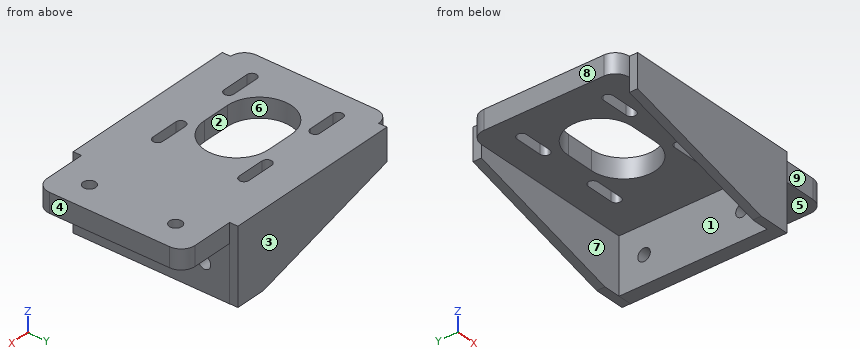
from build123d import *

# Parameters (mm, degrees)
F0_W      = 90
F0_H      = 53.2
F0_R      = 2.25
F1_DEPTH  = 3.5
F2_R      = 5
F3_W      = 5
F3_H      = 20
F4_DEPTH  = 26.6
F6_DEPTH  = 3
F8_DEPTH  = 3
F9_R      = 2.25
F10_DEPTH = 5


with BuildPart() as f1:
    # F0 (on Top) → F1 (new body, symmetric)
    with BuildSketch(Plane.XY):
        Rectangle(F0_W, F0_H)
        with BuildLine():
            ThreePointArc((-35.77, -17.25), (-37.52, -15.5), (-35.77, -13.75))
            Line((-35.77, -13.75), (-25.77, -13.75))
            ThreePointArc((-25.77, -13.75), (-24.02, -15.5), (-25.77, -17.25))
            Line((-25.77, -17.25), (-35.77, -17.25))
        make_face(mode=Mode.SUBTRACT)
        with BuildLine():
            Line((-4.77, -13.75), (5.23, -13.75))
            ThreePointArc((5.23, -13.75), (6.98, -15.5), (5.23, -17.25))
            Line((5.23, -17.25), (-4.77, -17.25))
            ThreePointArc((-4.77, -17.25), (-6.52, -15.5), (-4.77, -13.75))
        make_face(mode=Mode.SUBTRACT)
        with Locations((35, -15.5)):
            Circle(F0_R, mode=Mode.SUBTRACT)
        with BuildLine():
            ThreePointArc((-10.27, 11.5), (1.23, 0), (-10.27, -11.5))
            Line((-10.27, -11.5), (-20.27, -11.5))
            ThreePointArc((-20.27, -11.5), (-31.77, 0), (-20.27, 11.5))
            Line((-20.27, 11.5), (-10.27, 11.5))
        make_face(mode=Mode.SUBTRACT)
        with BuildLine():
            Line((-25.77, 13.75), (-35.77, 13.75))
            ThreePointArc((-35.77, 13.75), (-37.52, 15.5), (-35.77, 17.25))
            Line((-35.77, 17.25), (-25.77, 17.25))
            ThreePointArc((-25.77, 17.25), (-24.02, 15.5), (-25.77, 13.75))
        make_face(mode=Mode.SUBTRACT)
        with BuildLine():
            ThreePointArc((5.23, 17.25), (6.98, 15.5), (5.23, 13.75))
            Line((5.23, 13.75), (-4.77, 13.75))
            ThreePointArc((-4.77, 13.75), (-6.52, 15.5), (-4.77, 17.25))
            Line((-4.77, 17.25), (5.23, 17.25))
        make_face(mode=Mode.SUBTRACT)
        with Locations((35, 15.5)):
            Circle(F0_R, mode=Mode.SUBTRACT)
    extrude(amount=F1_DEPTH, both=True)

    # F2
    f2_edges = [f1.edges().sort_by_distance(p)[0] for p in [
        (-45, 26.6, 0),
        (-45, -26.6, 0),
        (45, -26.6, 0),
        (45, 26.6, 0),
    ]]
    fillet(f2_edges, radius=F2_R)

    # F3 (on Front) → F4 (join, symmetric)
    with BuildSketch(Plane.XZ):
        with Locations((22.5, -13.5)):
            Rectangle(F3_W, F3_H)
    extrude(amount=F4_DEPTH, both=True)

    # F5 (on face) → F6 (join)
    with BuildSketch(Plane.XZ.offset(26.6)):
        Polygon((13.8679239899, -23.5), (20, -23.5), (20, -3.5), (-40, -3.5), (-40, -8.5), align=None)
        Polygon((20, -23.5), (25, -23.5), (25, -3.5), (25, 3.5), (-40, 3.5), (-40, -3.5), (20, -3.5), align=None)
    extrude(amount=F6_DEPTH)

    # F7 (on face) → F8 (join)
    with BuildSketch(Plane(origin=(0, 26.6, 0), x_dir=(-1, 0, 0), z_dir=(0, 1, 0))):
        Polygon((-24.9622650445, 3.5), (-24.9622650445, -23.4764143825), (-20, -23.4764143825), (-20, -3.5), (40, -3.5), (40, 3.5), align=None)
        Polygon((-20, -3.5), (-20, -23.4764143825), (-13.8679249212, -23.4764143825), (40, -8.0235851929), (40, -3.5), align=None)
    extrude(amount=F8_DEPTH)

    # F9 (on face) → F10 (cut, through all)
    with BuildSketch(Plane.YZ.offset(25)):
        with Locations((-17.6, -13.5)):
            Circle(F9_R)
        with Locations((17.6, -13.5)):
            Circle(F9_R)
    extrude(amount=-F10_DEPTH, mode=Mode.SUBTRACT)


solid = f1.part
Read the model definition and answer for the solid it produces. Units are mm, in the model's axes. Face numbers are marked on the shaded views. A direction names the side the tool comes from. Round coordinates to 2 decimals unless told otherwise and drop trailing zeros. Loops run counter-clockwise (first coordinate to the right, second up) from the corner with the lowest first, then second, coordinate; pieces in that order, holes last.
Q1. Section C-C on x = -16 is taken. Write down the section's boundary in (y, z), and give its area (3 significant figures).
Q2. Consider probe 1 along Z at (x, y) = (23.15, -17.6); probe 2 along Y at (x, z) = (-5, -7.5); probe 3 along Y at (x, z) = (-25, 2.25). Determine where each line is inside the solid, lowest interval first.
Q3. Section A-A on y = 0 is taken. Write down the section's boundary in (x, z), and give its area (3 significant figures).
Q4. Section B-B on x = 19 is taken. Write down the section's boundary in (y, z).
Q5. Section D-D on y = -24 is taken. Write down the section's boundary in (x, z).
Q6. Each of these flat-tipped pins is pushed along its axis until it touches: pin 1 (16 mm diameter, centred on x = 31, z = -4.5, fed in from +Y); pin 2 (2.5 mm diameter, centred on y = 29, z = -5, fed in from -X); pin 3 (1.5 mm diameter, centred on x = 21, y = 28.5, fed in from -Z); pin 4 (6 mm diameter, centred on x = 34.5, y = 6.5, fed in from -Z). Where does it stop, or does it pass through?
Q7. Determine the mould class of the marked faces 1, 2, 3 and 4 for opening direction X: released by +X, released by -X, zero draft, split by the parting line, or undercut.
Q8. Which of the six approach directions +Z, -Z, +X, -X, +Y, -Y give full straight-line access (tool end or side, diameter ignored) to the marked faces 5, 6, 7, 8 and 9?
Output:
1. outline: (-29.6, -15.18) - (-26.6, -15.18) - (-26.6, -3.5) - (-11.5, -3.5) - (-11.5, 3.5) - (-29.6, 3.5) - close; (11.5, -3.5) - (26.6, -3.5) - (26.6, -14.91) - (29.6, -14.91) - (29.6, 3.5) - (11.5, 3.5) - close
1. area: 323 mm2
2. probe 1: z = -23.5 to -15.75, -11.25 to 3.5
2. probe 2: y = -29.6 to -26.6, 26.6 to 29.6
2. probe 3: y = -29.6 to -17.07, -13.93 to -10.48, 10.48 to 13.93, 17.07 to 29.6
3. outline: (-45, -3.5) - (-31.77, -3.5) - (-31.77, 3.5) - (-45, 3.5) - close; (1.23, -3.5) - (20, -3.5) - (20, -23.5) - (25, -23.5) - (25, -3.5) - (45, -3.5) - (45, 3.5) - (1.23, 3.5) - close
3. area: 499 mm2
4. outline: (-29.6, -23.5) - (-26.6, -23.5) - (-26.6, -3.5) - (26.6, -3.5) - (26.6, -23.48) - (29.6, -23.48) - (29.6, 3.5) - (-29.6, 3.5) - close
5. outline: (-44.39, -3.5) - (20, -3.5) - (20, -23.5) - (25, -23.5) - (25, -3.5) - (44.39, -3.5) - (44.39, 3.5) - (-44.39, 3.5) - close
6. pin 1: stops at y = 29.6
6. pin 2: stops at x = -40
6. pin 3: stops at z = -23.48
6. pin 4: stops at z = -3.5
7. face 1: released by -X
7. face 2: undercut
7. face 3: zero draft
7. face 4: released by +X
8. face 5: -Z, +X, +Y, -Y
8. face 6: +Z, -Z
8. face 7: -Z, -X
8. face 8: +Z, -Z, -X, +Y, -Y
8. face 9: +Z, -Z, +X, -Y
